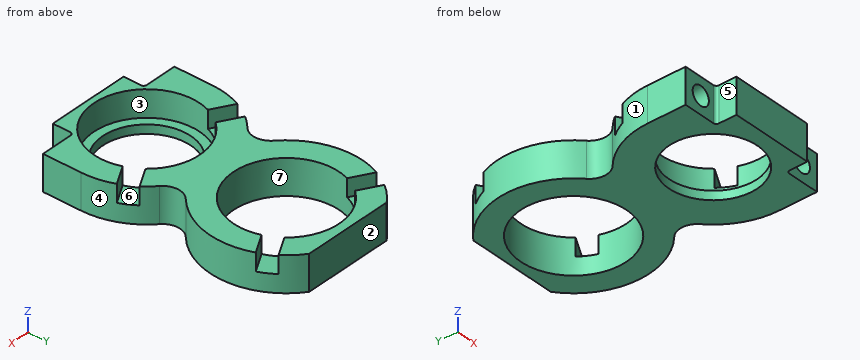
```python
from build123d import *

# Parameters (mm, degrees)
SKETCH_1_W          = 26
SKETCH_1_H          = 46.8
EXTRUDE_1_DEPTH     = 6
SKETCH_2_R          = 9
SKETCH_2_R_2        = 7.5
CUT_EXTRUDE_1_DEPTH = 54.872441935
SKETCH_3_W          = 26
SKETCH_3_H          = 2.5
CUT_EXTRUDE_2_DEPTH = 54.872441935
CHAMFER_1_SIZE      = 5
SKETCH_4_W          = 6
SKETCH_4_H          = 6
CUT_EXTRUDE_3_DEPTH = 3.5
SKETCH_5_R          = 1.6
CUT_EXTRUDE_4_DEPTH = 3
FILLET_1_R          = 0.5
SKETCH_6_OUTSIDE_W  = 38.344
SKETCH_6_OUTSIDE_H  = 56.644
CUT_EXTRUDE_5_DEPTH = 54.872441935
FILLET_2_R          = 3
SKETCH_7_R          = 9
CUT_EXTRUDE_6_DEPTH = 4.5
CUT_EXTRUDE_7_DEPTH = 3


with BuildPart() as part:
    # 草图1 → 凸台-拉伸1 (new body)
    with BuildSketch(Plane.XY):
        with Locations((13, 23.4)):
            Rectangle(SKETCH_1_W, SKETCH_1_H)
    extrude(amount=EXTRUDE_1_DEPTH)

    # 草图2 → 切除-拉伸1 (cut, through all)
    with BuildSketch(Plane.XY.offset(6)):
        with Locations((13, 36.3)):
            Circle(SKETCH_2_R)
        with Locations((13, 12.5)):
            Circle(SKETCH_2_R_2)
    extrude(amount=-CUT_EXTRUDE_1_DEPTH, mode=Mode.SUBTRACT)

    # 草图3 → 切除-拉伸2 (cut, through all)
    with BuildSketch(Plane.XY.offset(6)):
        with Locations((13, 1.25)):
            Rectangle(SKETCH_3_W, SKETCH_3_H)
    extrude(amount=-CUT_EXTRUDE_2_DEPTH, mode=Mode.SUBTRACT)

    # 倒角1
    chamfer_1_edges = [part.edges().sort_by_distance(p)[0] for p in [
        (0, 46.8, 3),
        (26, 46.8, 3),
    ]]
    chamfer(chamfer_1_edges, length=CHAMFER_1_SIZE)

    # 草图4 → 切除-拉伸3 (cut)
    with BuildSketch(Plane.XZ.offset(-2.5)):
        with Locations((3, 3)):
            Rectangle(SKETCH_4_W, SKETCH_4_H)
        with Locations((23, 3)):
            Rectangle(SKETCH_4_W, SKETCH_4_H)
    extrude(amount=-CUT_EXTRUDE_3_DEPTH, mode=Mode.SUBTRACT)

    # 草图5 → 切除-拉伸4 (cut)
    with BuildSketch(Plane.XZ.offset(-6)):
        with Locations(Location((3, 3, 0), (0, 0, 270))):
            Circle(SKETCH_5_R)
        with Locations(Location((23, 3, 0), (0, 0, 270))):
            Circle(SKETCH_5_R)
    extrude(amount=-CUT_EXTRUDE_4_DEPTH, mode=Mode.SUBTRACT)

    # 圆角1
    fillet_1_edges = [part.edges().sort_by_distance(p)[0] for p in [
        (6, 6, 3),
        (20, 6, 3),
    ]]
    fillet(fillet_1_edges, radius=FILLET_1_R)

    # 草图6 outside → 切除-拉伸5 (cut, through all)
    with BuildSketch(Plane.XY.offset(6)):
        with Locations((13, 24.65)):
            Rectangle(SKETCH_6_OUTSIDE_W, SKETCH_6_OUTSIDE_H)
        with BuildLine():
            Line((0, 12.5), (0, 6))
            Line((0, 6), (0, 0))
            Line((0, 0), (26, 0))
            Line((26, 0), (26, 6))
            Line((26, 6), (26, 12.5))
            ThreePointArc((26, 12.5), (23.886599408, 19.605065328), (18.233545643, 24.4))
            ThreePointArc((18.233545643, 24.4), (13, 49.3), (7.766454357, 24.4))
            ThreePointArc((7.766454357, 24.4), (2.113400592, 19.605065328), (0, 12.5))
        make_face(mode=Mode.SUBTRACT)
    extrude(amount=-CUT_EXTRUDE_5_DEPTH, mode=Mode.SUBTRACT)

    # 圆角2
    fillet_2_edges = [part.edges().sort_by_distance(p)[0] for p in [
        (18.233545643, 24.4, 3),
        (7.766454357, 24.4, 3),
    ]]
    fillet(fillet_2_edges, radius=FILLET_2_R)

    # 草图7 → 切除-拉伸6 (cut)
    with BuildSketch(Plane.XY.offset(6)):
        with Locations((13, 12.5)):
            Circle(SKETCH_7_R)
    extrude(amount=-CUT_EXTRUDE_6_DEPTH, mode=Mode.SUBTRACT)

    # 草图8 → 切除-拉伸7 (cut)
    with BuildSketch(Plane.XY.offset(6)):
        Polygon((5.159136754, 39.007700761), (6.659136754, 41.605776972), (1.007687062, 44.868642973), (-0.492312938, 42.270566762), align=None)
        Polygon((7.841745639, 13.746068736), (9.341745639, 16.344144947), (1.5, 20.871578903), (0, 18.273502692), align=None)
        Polygon((24.5, 20.871578903), (16.658254361, 16.344144947), (18.158254361, 13.746068736), (26, 18.273502692), align=None)
        Polygon((24.992312938, 44.868642973), (19.340863246, 41.605776972), (20.840863246, 39.007700761), (26.492312938, 42.270566762), align=None)
    extrude(amount=-CUT_EXTRUDE_7_DEPTH, mode=Mode.SUBTRACT)


solid = part.part
```
Model file for the job. Use its own axes, mm. Face numbers are marked on the shaded views. A direction names the side the tool comes from. Round coordinates to 2 decimals unless told otherwise and drop trailing zeros. Loops run counter-clockwise (first coordinate to the right, second up) from the corner with the lowest first, then second, coordinate; pieces in that order, holes last. Notation, with made-up numbers: M 16,11.25 L 34,11.25 A18 ccw 34,26.25 Z; hole C 6.5,22 d6. An arc over 180 degrees is marked long. Put each result on its own line as item: value. Start each with the question number.
Item 1: Drop flat-ended pins along their axis: P1, Ø9, axis at x = 13.5, y = 10, coming from the +Z side; P2, Ø1.6, axis at x = 3.5, z = 2.5, coming from the -Y side; P3, Ø4, axis at x = 13, y = 21, coming from the -Z side; P4, Ø3.5, axis at y = 4, z = 2, coming from the +X side. Give the stop position or say it passes through.
Item 2: Cut at C-C (y = 8.5). List the corners of the cut face in (x, z), then the cut area to 3 significant figures.
Item 3: Drill centre lines: line 1 along Y through (x, z) = (13, 1.3); line 2 along X through (y, z) = (12.5, 3.2); line 3 along Y through (x, z) = (13, 3.45). Where is each one in solid material? Low to high.
Item 4: Mould opens along X. For the marked faces 4, 5, 6 and 7 say: released by +X, released by -X, zero draft, split by the parting line, or undercut.
Item 5: 3-axis set-ups, long thin cutter, end or side, ignore diameter. For the marked faces 1, 2 and 3: which of +Z, -Z, +X, -X, +Y, -Y reach the whole face in a straight line?
Item 6: Cut at A-A (y = 36.3). List the corners of the cut face in (x, z).
Item 7: Cut at B-B (x = 13). List the corners of the cut face in (y, z), then the cut area to 3 significant figures.
Item 8: Cut at D-D (x = 3). List the corners of the cut face in (y, z).
Answer block:
1. P1: through
1. P2: y = 9
1. P3: z = 0
1. P4: x = 20.07
2. outline: M 0,0 L 6.66,0 L 6.66,1.5 L 4.94,1.5 L 4.94,6 L 0,6 Z; M 19.34,0 L 26,0 L 26,6 L 21.06,6 L 21.06,1.5 L 19.34,1.5 Z; hole C 3,3 d3.2; hole C 23,3 d3.2
2. area: 48.3 mm2
3. line 1: 2.5 to 5, 20 to 27.3, 45.3 to 46.8
3. line 2: 0 to 4, 22 to 26
3. line 3: 2.5 to 3.5, 21.5 to 27.3, 45.3 to 46.8
4. face 4: released by +X
4. face 5: released by -X
4. face 6: undercut
4. face 7: undercut
5. face 1: +Z, -Z, -X
5. face 2: +Z, -Z, +X, -X, +Y
5. face 3: +Z
6. outline: M 0,0 L 4,0 L 4,6 L 0,6 Z; M 22,0 L 26,0 L 26,6 L 22,6 Z
7. outline: M 2.5,0 L 5,0 L 5,1.5 L 3.5,1.5 L 3.5,6 L 2.5,6 Z; M 20,0 L 27.3,0 L 27.3,6 L 21.5,6 L 21.5,1.5 L 20,1.5 Z; M 45.3,0 L 46.8,0 L 46.8,6 L 45.3,6 Z
7. area: 54.3 mm2
8. outline: M 6,0 L 20.81,0 L 20.81,6 L 20.01,6 L 20.01,3 L 16.54,3 L 16.54,6 L 6,6 L 6,4.6 L 9,4.6 L 9,1.4 L 6,1.4 Z; M 27.99,0 L 44.61,0 L 44.61,6 L 43.72,6 L 43.72,3 L 40.25,3 L 40.25,6 L 27.99,6 Z
